Can you work these out from the model? Positions are in its coordinate system, mm. A direction names the side the tool comes from. Coordinates: 2 decimals unless noted, no trailing zeros. Loops run counter-clockwise (first coordinate to the right, second up) from the corner with the lowest first, then second, coordinate; pieces in that order, holes last.
Autodesk Inventor part; units mm, degrees
ref_plane "Plano de trabalho1" through (0, -17.5, 88.75) normal (1, 0, 0) x (0, 0, -1)
ref_plane "YZ Plane" through (0, 0, 0) normal (1, 0, 0) x (0, 1, 0)
ref_plane "XZ Plane" through (0, 0, 0) normal (0, 1, 0) x (-1, 0, 0)
sketch "Esboço1" plane through (0, 0, 0) normal (0, 1, 0) x (-1, 0, 0)
  line L0 (-25, 76.25) -> (25, 76.25)
  line L1 (25, 76.25) -> (25, -76.25)
  line L2 (25, -76.25) -> (-25, -76.25)
  line L3 (-25, -76.25) -> (-25, 76.25)
  line L4 (-25, 76.25) -> (25, -76.25) construction
  line L5 (25, 76.25) -> (-25, -76.25) construction
  line L6 (0, 88.75) -> (0, 63.75) construction
  line L7 (-25, 88.75) -> (-25, 63.75)
  line L8 (25, 63.75) -> (25, 88.75)
  arc A0 (25, 88.75) -> (-25, 88.75) centre (0, 88.75) ccw
  arc A1 (-25, 63.75) -> (25, 63.75) centre (0, 63.75) ccw
  point P0 (0, 0)
  point P1 (0, 76.25)
  point P2 (0, 113.75)
  dimension "d1" = 25
  dimension "d2" = 50
  dimension "d3" = 190
extrude "Extrusão1" add sketch "Esboço1" along normal mid plane 35 contours L7 A0 L8 L0 | L0 L1 A1 L3
extrude "Extrusão2" add sketch "Esboço1" along normal mid plane 10 contours A1 L1 L2 L3
ref_plane "Plano de trabalho1" through (0, -17.5, 88.75) normal (1, 0, 0) x (0, 0, -1)
sketch "Esboço3" plane through (0, -17.5, 88.75) normal (1, 0, 0) x (0, 0, -1)
  circle A0 centre (140, 68) radius 25
  line L0 (165, 12.5) -> (165, 22.5)
  line L1 (165, 12.5) -> (25, 12.5)
  point P0 (88.75, 17.5)
  dimension "d8" = 50
  dimension "d9" = 55.5
extrude "Extrusão3" add sketch "Esboço3" along normal mid plane 30
sketch "Esboço5" plane through (0, -17.5, 88.75) normal (1, 0, 0) x (0, 0, -1)
  circle A0 centre (140, 68) radius 25
  line L0 (165, 68) -> (165, 22.5)
  line L1 (165, 22.5) -> (11.9907, 22.5)
  line L2 (11.9907, 22.5) -> (11.9907, 30.5)
  line L3 (11.9907, 22.5) -> (165, 22.5)
  line L4 (115, 68) -> (165, 68)
  line L5 (11.9907, 30.5) -> (97, 30.5)
  line L6 (115, 48.5) -> (115, 68)
  line L7 (165, 22.5) -> (25, 22.5)
  arc A1 (97, 30.5) -> (115, 48.5) centre (97, 48.5) ccw
  line L8 (165, 22.5) -> (165, 12.5)
  point P0 (88.75, 17.5)
  dimension "d14" = 8
  dimension "d15" = 18
extrude "Extrusão4" add sketch "Esboço5" along normal mid plane 10 contours L0 L1 L2 L5 A1 L6 A0
sketch "Esboço6" plane through (15, 50.5, -51.25) normal (1, 0, 0) x (0, 0, -1)
  circle A0 centre (0, 0) radius 25
  point P0 (-51.25, -50.5)
hole "Furo1" at (15, 50.5, -51.25) direction (-1, 0, 0) diameter 25 end through all
sketch "Esboço7" plane through (0, 17.5, 0) normal (0, 1, 0) x (1, 0, 0)
  line L0 (25, -88.75) -> (25, -63.75)
  arc A0 (25, -63.75) -> (-25, -63.75) centre (0, -63.75) ccw
  line L1 (-25, -63.75) -> (-25, -88.75)
  arc A1 (-25, -88.75) -> (25, -88.75) centre (0, -88.75) ccw
  line L2 (10, -88.75) -> (10, -63.75)
  arc A2 (10, -63.75) -> (-10, -63.75) centre (0, -63.75) ccw
  line L3 (-10, -63.75) -> (-10, -88.75)
  arc A3 (-10, -88.75) -> (10, -88.75) centre (0, -88.75) ccw
  point P0 (0, 0)
  dimension "d25" = 20
extrude "Extrusão5" cut sketch "Esboço7" against normal through all contours A3 L3 A2 L2
properties part number "Peça teste 6"
Item 1: Suppose I cut it at A-A, the plane x = -2.5. Please give me the cut outline in (y, z).
Results are:
outline: (-17.5, 38.88) - (-5, 38.88) - (-5, -76.25) - (50.5, -76.25) arc R25 ccw to (50.5, -26.25) - (31, -26.25) arc R18 cw to (13, -8.25) - (13, 38.88) - (17.5, 38.88) - (17.5, 54.07) - (-17.5, 54.07) - close; (-17.5, 98.43) - (17.5, 98.43) - (17.5, 113.62) - (-17.5, 113.62) - close; hole circle Ø25 at (50.5, -51.25)
Item 2: We'd pull the mould along X, two halves only. Please class faces 5 (the face through (0.55, -0.245, 113.744)), 6 (the face through (-0.22, 0.245, 98.748)), 7 (the face through (15, 56.4, -39.8)): +X half, -X half, draft (parallel to the pull), parting line (faces both ways), or undercut.
Results are:
face 5: parting line
face 6: undercut
face 7: +X half
Item 3: Suppose I cut it at B-B, the plane y = 7. Please give me the cut outline in (x, z).
Results are:
outline: (-25, 63.75) arc R25 ccw to (-5, 39.26) - (-5, -76.25) - (5, -76.25) - (5, 39.26) arc R25 ccw to (25, 63.75) - (25, 88.75) arc R25 ccw to (-25, 88.75) - close; hole (-10, 63.75) arc R10 ccw to (10, 63.75) - (10, 88.75) arc R10 ccw to (-10, 88.75) - close
Item 4: I'm going to push flat-ended pins straight in: P1, Ø6, axis at x = 15, z = -26, coming from the +Y side; P2, Ø13.5, axis at y = 25, z = -19.5, coming from the -X side; P3, Ø3, axis at x = 1.5, z = 17.5, coming from the +Y side; P4, Ø6, axis at x = -5, z = 93.5, coming from the -Y side. Where does each tip first touch, or does it pass through?
Results are:
P1: stops at y = 61.9
P2: stops at x = -5
P3: stops at y = 13
P4: passes through
Item 5: On a 3-axis mill with a long thin cutter (end or side, diameter ignored), from which of +Z, -Z, +X, -X, +Y, -Y can I reach the whole of each face in a straight line? I mean faces 1 (the face through (-15, 56.4, -39.8)), 2 (the face through (0.21, 75.287, -47.995)), 3 (the face through (-10, 0, 76)), 4 (the face through (-0.07, 18.413, -21.117)). Say none if no direction works.
Results are:
face 1: +Z, -Z, -X, +Y
face 2: none
face 3: +Y, -Y
face 4: +X, -X, +Y
Item 6: Suppose I cut it at C-C, the plane y = 58. Please give me the cut outline in (x, z).
Results are:
outline: (-15, -75.1) - (15, -75.1) - (15, -61.25) - (-15, -61.25) - close; (-15, -41.25) - (15, -41.25) - (15, -27.4) - (-15, -27.4) - close
Item 7: Suppose I cut it at D-D, the plane x = -12. Please give me the cut outline in (y, z).
Results are:
outline: (-17.5, 41.82) - (-5, 41.82) - (-5, -76.25) - (5, -76.25) - (5, 41.82) - (17.5, 41.82) - (17.5, 110.68) - (-17.5, 110.68) - close; circle Ø50 at (50.5, -51.25); hole circle Ø25 at (50.5, -51.25)
Item 8: I need wall thicknesses on line 1 along Y through (x, z) = (7.5, -51.25); line 2 along Y through (x, z) = (4, -51); line 3 along Z through (x, y) = (-6.5, 50.5). Which ranges of each line are inside material? Lowest first, please.
Results are:
line 1: y = -5 to 5, 25.5 to 38, 63 to 75.5
line 2: y = -5 to 38, 63 to 75.5
line 3: z = -76.25 to -63.75, -38.75 to -26.25
